```python
from build123d import *

# Parameters (mm, degrees)
F1_DEPTH = 12.7
F3_D     = 3.175
F4_D     = 6.35
F6_D     = 4.4958
F8_D     = 3.4544
F10_D    = 3.4544


with BuildPart() as f1:
    # F0 (on Front) → F1 (new body)
    with BuildSketch(Plane.XZ):
        Polygon((-37.8843045536, 62.8095008674), (-47.3331045536, 62.8095008674), (-47.3331045536, 12.0095008674), (22.1612954464, 12.0095008674), (22.1612954464, 62.8095008674), (12.7124954464, 62.8095008674), (12.7124954464, 31.0595008674), (-37.8843045536, 31.0595008674), align=None)
    extrude(amount=F1_DEPTH)

    # F3 (through all)
    with Locations(Plane.XZ.offset(12.7)):
        with Locations((-28.2831045536, 31.0595008674), (-18.7581045536, 31.0595008674), (3.0985954464, 31.0595008674)):
            Hole(F3_D / 2)

    # F4 (through all)
    with Locations(Plane.XZ.offset(12.7)):
        with Locations((-7.6456045536, 31.0595008674)):
            Hole(F4_D / 2)

    # F6 (through all)
    with Locations(Plane.XZ.offset(12.7)):
        with Locations((-42.5706045536, 56.4595008674), (17.3987954464, 56.4595008674)):
            Hole(F6_D / 2)

    # F8 (through all)
    with Locations(Plane.XY.offset(31.0595008674)):
        with Locations((-34.6331045536, -6.35)):
            Hole(F8_D / 2)

    # F10 (through all)
    with Locations(Plane.XY.offset(31.0595008674)):
        with Locations((9.4612954464, -6.35)):
            Hole(F10_D / 2)


solid = f1.part
```
The model under review builds one solid part; all positions refer to its coordinate system, in mm. A direction names the side the tool comes from. Round coordinates to 2 decimals unless told otherwise and drop trailing zeros. Order: outer loops, then holes, each group sorted by start corner. A loop starts at its lowest first (then second) coordinate and runs counter-clockwise, first axis right, second up. Notation, with made-up numbers: (71, 28.25) -> (85, 28.25) arc R32 cw to (85, 57.25) -> close; hole circle Ø3 at (-1.5, -0.5). An arc over 180 degrees is marked (long way). Use a Markdown table: item, result.
Q1. Clearance check with a flat-ended pin moving along its axis: P1, Ø3, axis at x = -23.5, y = -4, coming from the +Z side. State where the tip first meets the part, or that it passes through.
Values:
| item | result |
|---|---|
| P1 | stops at z = 31.06 |
Q2. We need section A-A on y = -6.35. State how many separate pieces and enclosed holes the cut face has, then the cut area to 3 significant figures.
Values:
| item | result |
|---|---|
| separate pieces | 3 |
| enclosed holes | 2 |
| area | 1,730 mm^2 |
Q3. For line 1 (X direction, y = -6.5, z = 35); line 2 (X direction, y = -8.75, z = 56); line 3 (X direction, y = -5.75, z = 25), list the stretches that pass through material, from the lowest coordinate up.
Values:
| item | result |
|---|---|
| line 1 | x = -47.33 to -37.88, 12.71 to 22.16 |
| line 2 | x = -47.33 to -44.77, -40.37 to -37.88, 12.71 to 15.2, 19.6 to 22.16 |
| line 3 | x = -47.33 to -36.25, -33.01 to 7.84, 11.08 to 22.16 |
Q4. We need section D-D on x = -24. Write out the cut boundary in (y, z).
Values:
| item | result |
|---|---|
| outline | (-12.7, 12.01) -> (0, 12.01) -> (0, 31.06) -> (-12.7, 31.06) -> close |
Q5. We need section B-B on z = 52. Write out the cut boundary in (x, y).
Values:
| item | result |
|---|---|
| outline | (-47.33, -12.7) -> (-37.88, -12.7) -> (-37.88, 0) -> (-47.33, 0) -> close; (12.71, -12.7) -> (22.16, -12.7) -> (22.16, 0) -> (12.71, 0) -> close |
Q6. Tool access review of faces 4 (the flat face through (-47.333, -6, 38)), 5 (the flat face through (-33, -5, 31.06)): name each direction out of +Z, -Z, +X, -X, +Y, -Y from which nothing blocks a thin tool from reaching the whole face with its end or side.
Values:
| item | result |
|---|---|
| face 4 | +Z, -Z, -X, +Y, -Y |
| face 5 | +Z, +Y, -Y |
Q7. Mouldability with a two-part tool opening along Z and no side actions: class faces 1 (the flat face through (-37.884, -6, 47)), 2 (the flat face through (-14, -6, 31.06)), 3 (the cylindrical face through (-40.79, -6.26, 55.09)) as +Z half, -Z half, draft (parallel to the pull), parting line (faces both ways), or undercut.
Values:
| item | result |
|---|---|
| face 1 | draft |
| face 2 | +Z half |
| face 3 | undercut |
